```python
from build123d import *

# Parameters (mm, degrees)
BOSS_EXTRU_1_DEPTH = 3


with BuildPart() as part:
    # Esquisse1 → Boss.-Extru.1 (new body)
    with BuildSketch(Plane.XY):
        with BuildLine():
            Line((-220, 295), (-30, 295))
            ThreePointArc((-30, 295), (-22.928932188, 297.928932188), (-20, 305))
            Line((-20, 305), (-20, 335))
            Line((-20, 335), (20, 335))
            Line((20, 335), (20, 305))
            ThreePointArc((20, 305), (22.928932188, 297.928932188), (30, 295))
            Line((30, 295), (220, 295))
            ThreePointArc((220, 295), (234.142135624, 289.142135624), (240, 275))
            Line((240, 275), (240, -125))
            ThreePointArc((240, -125), (234.142135624, -139.142135624), (220, -145))
            Line((220, -145), (-220, -145))
            ThreePointArc((-220, -145), (-234.142135624, -139.142135624), (-240, -125))
            Line((-240, -125), (-240, 275))
            ThreePointArc((-240, 275), (-234.142135624, 289.142135624), (-220, 295))
        make_face()
    extrude(amount=BOSS_EXTRU_1_DEPTH)


solid = part.part
```
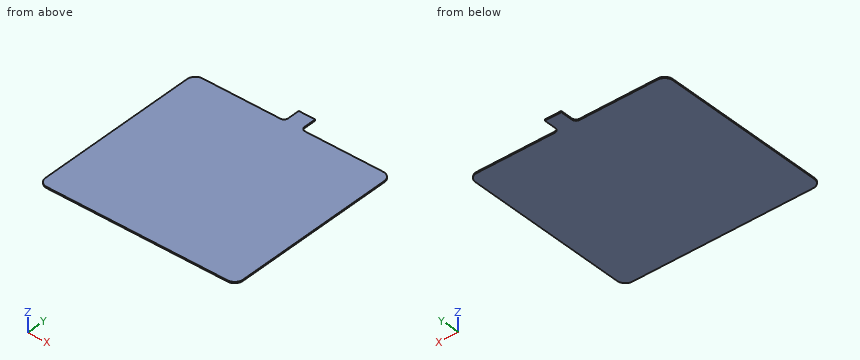
Part model, mm, in its own coordinate system. Round coordinates to 2 decimals unless told otherwise and drop trailing zeros. Order: outer loops, then holes, each group sorted by start corner. A loop starts at its lowest first (then second) coordinate and runs counter-clockwise, first axis right, second up. Notation, with made-up numbers: M 68,-12 L 123,-12 A19 cw 123,-2 Z; hole C 39,19 d1. An arc over 180 degrees is marked long. Answer in a Markdown table with one row per item. Add a question column.
Q1. Wall check: L1, parallel to Y at x = -75, z = 0.3. Give the ranges that are in metal, low to high. Write a range as from..to.
Q2. Cut at A-A on z = 1.6. Give the cut face in (x, y).
Q3. Cut at B-B on x = -83. Give the cut face in (y, z), and give its area (3 significant figures).
Q4. Pin check, flat tips, straight feed: pin 1 (0.9 mm diameter, centred on x = 95, z = 1, fed in from +Y); pin 2 (1 mm diameter, centred on y = 281, z = 1.5, fed in from -X); pin 3 (1.5 mm diameter, centred on y = 326.5, z = 2, fed in from -X). Stop position of each tip, or through.
Established:
| question | item | result |
|---|---|---|
| 1 | L1 | y = -145..295 |
| 2 | outline | M -240,-125 A20 ccw -220,-145 L 220,-145 A20 ccw 240,-125 L 240,275 A20 ccw 220,295 L 30,295 A10 cw 20,305 L 20,335 L -20,335 L -20,305 A10 cw -30,295 L -220,295 A20 ccw -240,275 Z |
| 3 | outline | M -145,0 L 295,0 L 295,3 L -145,3 Z |
| 3 | area | 1,320 mm2 |
| 4 | pin 1 | stops at y = 295 |
| 4 | pin 2 | stops at x = -239.23 |
| 4 | pin 3 | stops at x = -20 |
